The listing builds one solid part. Answer for the finished solid, in the listing's coordinates (mm). Coordinates: 2 decimals unless noted, no trailing zeros. Order: outer loops, then holes, each group sorted by start corner. A loop starts at its lowest first (then second) coordinate and runs counter-clockwise, first axis right, second up. Notation, with made-up numbers: (-16.75, 8.5) -> (10.25, 8.5) arc R25 ccw to (10.25, 27.5) -> close; hole circle Ø1 at (-10, -6.5). An arc over 180 degrees is marked (long way). Answer in a Markdown table with one row per item. Add a question column.
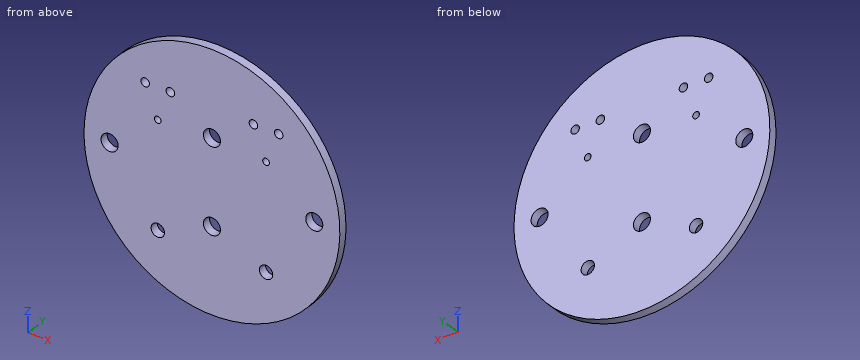
```python
from build123d import *

# Parameters (mm, degrees)
SKETCH1_R           = 47.625
BOSS_EXTRUDE1_DEPTH = 3.175
SKETCH2_R           = 3.175
CUT_EXTRUDE1_DEPTH  = 263.398
SKETCH3_R           = 3.175
CUT_EXTRUDE2_DEPTH  = 25.4
SKETCH4_R           = 1.5875
SKETCH4_R_2         = 1.25
CUT_EXTRUDE3_DEPTH  = 50.8
CUT_EXTRUDE4_START  = -3.175
SKETCH5_R           = 1.984375
CUT_EXTRUDE4_DEPTH  = 50.8
SKETCH6_R           = 2.4892
CUT_EXTRUDE5_DEPTH  = 25.4


with BuildPart() as part:
    # Sketch1 → Boss-Extrude1 (new body)
    with BuildSketch(Plane(origin=(0, 0, 0), x_dir=(1, 0, 0), z_dir=(0, 1, 0))):
        with Locations(Location((0, 0, 0), (0, 0, 270))):
            Circle(SKETCH1_R)
    extrude(amount=BOSS_EXTRUDE1_DEPTH)

    # Sketch2 → Cut-Extrude1 (cut)
    with BuildSketch(Plane(origin=(-55.039702575, 231.775, -116.088398355), x_dir=(-1, 0, 0), z_dir=(0, 1, 0))):
        with Locations(Location((-93.139702575, 116.088398355, 0), (0, 0, 90))):
            Circle(SKETCH2_R)
        with Locations(Location((-16.939702575, 116.088398355, 0), (0, 0, 90))):
            Circle(SKETCH2_R)
    extrude(amount=-CUT_EXTRUDE1_DEPTH, mode=Mode.SUBTRACT)

    # Sketch3 → Cut-Extrude2 (cut)
    with BuildSketch(Plane(origin=(-28.264398128, -3.175, -82.371298873), x_dir=(1, 0, 0), z_dir=(0, -1, 0))):
        with Locations(Location((28.264398128, 98.246298873, 0), (0, 0, 90))):
            Circle(SKETCH3_R)
        with Locations(Location((28.264398128, 66.496298873, 0), (0, 0, 90))):
            Circle(SKETCH3_R)
    extrude(amount=-CUT_EXTRUDE2_DEPTH, mode=Mode.SUBTRACT)

    # Sketch4 → Cut-Extrude3 (cut)
    with BuildSketch(Plane(origin=(-28.264398128, -3.175, -82.371298873), x_dir=(-1, 0, 0), z_dir=(0, -1, 0))):
        with Locations(Location((-3.404148128, -108.914298873, 0), (0, 0, 270))):
            Circle(SKETCH4_R)
        with Locations(Location((-12.802148128, -108.914298873, 0), (0, 0, 270))):
            Circle(SKETCH4_R)
        with Locations(Location((-43.726648128, -108.914298873, 0), (0, 0, 270))):
            Circle(SKETCH4_R)
        with Locations(Location((-53.124648128, -108.914298873, 0), (0, 0, 270))):
            Circle(SKETCH4_R)
        with Locations(Location((-8.103148128, -97.230298873, 0), (0, 0, 270))):
            Circle(SKETCH4_R_2)
        with Locations(Location((-48.425648128, -97.230298873, 0), (0, 0, 270))):
            Circle(SKETCH4_R_2)
    extrude(amount=-CUT_EXTRUDE3_DEPTH, mode=Mode.SUBTRACT)

    # Sketch5 → Cut-Extrude4 (cut)
    with BuildSketch(Plane(origin=(-28.264398128, -3.175, -82.371298873), x_dir=(1, 0, 0), z_dir=(0, -1, 0)).offset(CUT_EXTRUDE4_START)):
        with Locations(Location((8.103148128, 57.606298873, 0), (0, 0, 90))):
            Circle(SKETCH5_R)
        with Locations(Location((48.425648128, 57.606298873, 0), (0, 0, 90))):
            Circle(SKETCH5_R)
    extrude(amount=-CUT_EXTRUDE4_DEPTH, mode=Mode.SUBTRACT)

    # Sketch6 → Cut-Extrude5 (cut)
    with BuildSketch(Plane(origin=(-28.264398128, 3.175, -82.371298873), x_dir=(1, 0, 0), z_dir=(0, 1, 0))):
        with Locations(Location((8.103148128, -57.606298873, 0), (0, 0, 270))):
            Circle(SKETCH6_R)
        with Locations(Location((48.425648128, -57.606298873, 0), (0, 0, 270))):
            Circle(SKETCH6_R)
    extrude(amount=-CUT_EXTRUDE5_DEPTH, mode=Mode.SUBTRACT)


solid = part.part
```
Q1. Given pin 1 (4 mm diameter, centred on x = 24.86, z = 26.54, fed in from -Y), flat-ended and moving along its own axis, determine where the tip first touches the part or whether it passes through.
Q2. A cutting plane is placed at B-B (x = 2). Determine the outline of the cut face in (y, z) (3 decimals).
Q3. A cutting plane is placed at A-A (z = 0). Determine the outline of the cut face in (x, y) (3 decimals).
Q4. Straight lines are drawn through the part: line 1 (X direction, y = 0.75, z = 0) (3 decimals); line 2 (X direction, y = 1.45, z = -26); line 3 (Z direction, x = 1, y = 1.25). For each, find the intervals that lie inside material, in ascending order.
Q5. A cutting plane is placed at C-C (x = 38.1). Determine the outline of the cut face in (y, z) (3 decimals).
Q6. A cutting plane is placed at D-D (y = 1.05). State how many separate pieces and enclosed holes the cut face has, then the cut area to 3 significant figures.
Returned:
| question | item | result |
|---|---|---|
| 1 | pin 1 | stops at y = 0 |
| 2 | outline | (0, -47.583) -> (3.175, -47.583) -> (3.175, -18.341) -> (0, -18.341) -> close; (0, -13.409) -> (3.175, -13.409) -> (3.175, 13.409) -> (0, 13.409) -> close; (0, 18.341) -> (3.175, 18.341) -> (3.175, 47.583) -> (0, 47.583) -> close |
| 3 | outline | (-47.625, 0) -> (-41.275, 0) -> (-41.275, 3.175) -> (-47.625, 3.175) -> close; (-34.925, 0) -> (34.925, 0) -> (34.925, 3.175) -> (-34.925, 3.175) -> close; (41.275, 0) -> (47.625, 0) -> (47.625, 3.175) -> (41.275, 3.175) -> close |
| 4 | line 1 | x = -47.625 to -41.275, -34.925 to 34.925, 41.275 to 47.625 |
| 4 | line 2 | x = -39.9 to -22.32, -18 to 18, 22.32 to 39.9 |
| 4 | line 3 | z = -47.61 to -18.89, -12.86 to 12.86, 18.89 to 47.61 |
| 5 | outline | (0, -28.575) -> (3.175, -28.575) -> (3.175, -3.175) -> (0, -3.175) -> close; (0, 3.175) -> (3.175, 3.175) -> (3.175, 28.575) -> (0, 28.575) -> close |
| 6 | separate pieces | 1 |
| 6 | enclosed holes | 12 |
| 6 | area | 6,920 mm² |
